Geometry: final body of the model. Coordinates: model frame, mm. Face numbers are marked on the shaded views. A direction names the side the tool comes from. Round coordinates to 2 decimals unless told otherwise and drop trailing zeros. Loops run counter-clockwise (first coordinate to the right, second up) from the corner with the lowest first, then second, coordinate; pieces in that order, holes last. Notation, with made-up numbers: (83.25, -22.5) -> (99.25, -22.5) arc R29 ccw to (99.25, 3.5) -> close; hole circle Ø4 at (54.25, -4). An arc over 180 degrees is marked (long way). Answer in a Markdown table with one row per item.
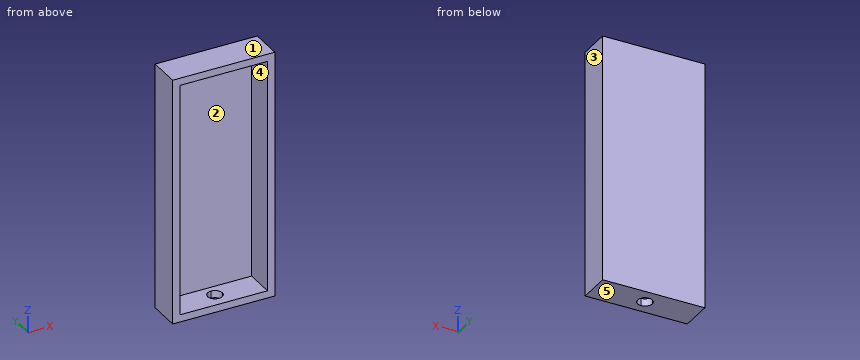
```python
from build123d import *

# Parameters (mm, degrees)
F0_W     = 6.35
F0_H     = 6.35
F1_DEPTH = 27.94
F2_W     = 88.9
F2_H     = 2.54
F3_DEPTH = 209.55
F5_DEPTH = 25.4


with BuildPart() as f1:
    # F0 (on Front) → F1 (new body)
    with BuildSketch(Plane.XZ):
        Polygon((-90.272094512, -40.0971807539), (-90.272094512, 163.1028192461), (-96.622094512, 163.1028192461), (-96.622094512, -46.4471807539), (-14.072094512, -46.4471807539), (-14.072094512, -40.0971807539), align=None)
        with Locations((-93.447094512, 166.2778192461)):
            Rectangle(F0_W, F0_H)
        Polygon((-90.272094512, 169.4528192461), (-90.272094512, 163.1028192461), (-14.072094512, 163.1028192461), (-14.072094512, -40.0971807539), (-7.722094512, -40.0971807539), (-7.722094512, 169.4528192461), align=None)
        with Locations((-10.897094512, -43.2721807539)):
            Rectangle(F0_W, F0_H)
    extrude(amount=F1_DEPTH)

    # F2 (on face) → F3 (join)
    with BuildSketch(Plane(origin=(0, 0, -46.4471807539), x_dir=(1, 0, 0), z_dir=(0, 0, -1))):
        with Locations((-52.172094512, 1.27)):
            Rectangle(F2_W, F2_H)
    extrude(amount=-F3_DEPTH)

    # F4 (on face) → F5 (cut)
    with BuildSketch(Plane(origin=(0, 0, -46.4471807539), x_dir=(1, 0, 0), z_dir=(0, 0, -1))):
        with BuildLine():
            Line((-58.522094512, 13.97), (-52.172094512, 13.97))
            Line((-52.172094512, 13.97), (-52.172094512, 20.32))
            ThreePointArc((-52.172094512, 20.32), (-56.6622225725, 18.4601280605), (-58.522094512, 13.97))
        make_face()
        with BuildLine():
            Line((-52.172094512, 13.97), (-45.822094512, 13.97))
            ThreePointArc((-45.822094512, 13.97), (-47.6819664515, 18.4601280605), (-52.172094512, 20.32))
            Line((-52.172094512, 20.32), (-52.172094512, 13.97))
        make_face()
        with BuildLine():
            ThreePointArc((-52.172094512, 7.62), (-47.6819664515, 9.4798719395), (-45.822094512, 13.97))
            Line((-45.822094512, 13.97), (-52.172094512, 13.97))
            Line((-52.172094512, 13.97), (-52.172094512, 7.62))
        make_face()
        with BuildLine():
            Line((-52.172094512, 7.62), (-52.172094512, 13.97))
            Line((-52.172094512, 13.97), (-58.522094512, 13.97))
            ThreePointArc((-58.522094512, 13.97), (-56.6622225725, 9.4798719395), (-52.172094512, 7.62))
        make_face()
    extrude(amount=-F5_DEPTH, mode=Mode.SUBTRACT)


solid = f1.part
```
Item 1: Line query: probe 1 along X at (y, z) = (-9.75, -19); probe 2 along Z at (x, y) = (-47.5, -3.5); probe 3 along Y at (x, z) = (-54, -12.5). Output: solid intervals per line, ascending. Write a range as [from, to].
Answer:
| item | result |
|---|---|
| probe 1 | x = [-96.62, -90.27], [-14.07, -7.72] |
| probe 2 | z = [-46.45, -40.1], [163.1, 169.45] |
| probe 3 | y = [-2.54, 0] |
Item 2: Cut plane D-D (y = -10.5). Output: boundary loops of the cut face in (x, z).
Answer:
| item | result |
|---|---|
| outline | (-96.62, -46.45) -> (-57.49, -46.45) -> (-57.49, -40.1) -> (-90.27, -40.1) -> (-90.27, 163.1) -> (-14.07, 163.1) -> (-14.07, -40.1) -> (-46.85, -40.1) -> (-46.85, -46.45) -> (-7.72, -46.45) -> (-7.72, 169.45) -> (-96.62, 169.45) -> close |
Item 3: Cut plane C-C (z = -25). Output: boundary loops of the cut face in (x, y), then the cut area to 3 significant figures.
Answer:
| item | result |
|---|---|
| outline | (-96.62, -27.94) -> (-90.27, -27.94) -> (-90.27, -2.54) -> (-14.07, -2.54) -> (-14.07, -27.94) -> (-7.72, -27.94) -> (-7.72, 0) -> (-96.62, 0) -> close |
| area | 548 mm² |
Item 4: Reachability of the marked faces 1 and 2 from +Z, -Z, +X, -X, +Y, -Y: full face, straight path, thin tool, end or side. Return the list, or none.
Answer:
| item | result |
|---|---|
| face 1 | +Z, +X, -X, +Y, -Y |
| face 2 | -Y |
Item 5: Cut plane A-A (x = -61.5). Output: boundary loops of the cut face in (y, z).
Answer:
| item | result |
|---|---|
| outline | (-27.94, -46.45) -> (0, -46.45) -> (0, 169.45) -> (-27.94, 169.45) -> (-27.94, 163.1) -> (-2.54, 163.1) -> (-2.54, -40.1) -> (-27.94, -40.1) -> close |
Item 6: Cut plane B-B (y = -25.25). Output: boundary loops of the cut face in (x, z).
Answer:
| item | result |
|---|---|
| outline | (-96.62, -46.45) -> (-7.72, -46.45) -> (-7.72, 169.45) -> (-96.62, 169.45) -> close; hole (-90.27, -40.1) -> (-14.07, -40.1) -> (-14.07, 163.1) -> (-90.27, 163.1) -> close |
Item 7: Pin query (flat end, axial travel): pin 1 Ø12 at (x, z) = (-70, 6.5) entering from -Y. Return the tip coordinate at first contact, or that it passes through.
Answer:
| item | result |
|---|---|
| pin 1 | stops at y = -2.54 |
Item 8: Draft query along Z for the marked faces 3, 4 and 5. Return one class per face: pulls with the +Z half, pulls with the -Z half, needs draft (parallel to the pull), parting line crosses it, or undercut.
Answer:
| item | result |
|---|---|
| face 3 | needs draft |
| face 4 | undercut |
| face 5 | pulls with the -Z half |
